from build123d import *

# Parameters (mm, degrees)
F1_DEPTH = 38.1
F3_DEPTH = 12.7
F5_DEPTH = 12.7
F6_DEPTH = 25.4
F8_DEPTH = 12.7


with BuildPart() as f1:
    # F0 (on Front) → F1 (new body)
    with BuildSketch(Plane.XZ):
        Polygon((0, 12.7), (0, 0), (25.4, 0), (25.4, 38.1), (12.7, 38.1), (12.7, 12.7), align=None)
    extrude(amount=F1_DEPTH)

    # F2 (on face) → F3 (cut)
    with BuildSketch(Plane(origin=(12.7, 0, 0), x_dir=(0, -1, 0), z_dir=(-1, 0, 0))):
        Polygon((38.1, 38.1), (25.4, 38.1), (38.1, 12.7), align=None)
    extrude(amount=-F3_DEPTH, mode=Mode.SUBTRACT)

    # F4 (on face) → F5 (join)
    with BuildSketch(Plane.XY.offset(12.7)):
        Polygon((0, -38.1), (12.7, -38.1), (0, -31.632963568), align=None)
    extrude(amount=F5_DEPTH)

    # F6 (cut): a face of the model
    f6_faces = [f1.faces().sort_by_distance(p)[0] for p in [
        (6.35, -34.866481784, 19.05),
    ]]
    extrude(f6_faces, amount=-F6_DEPTH, mode=Mode.SUBTRACT)

    # F7 (on face) → F8 (cut)
    with BuildSketch(Plane.XY.offset(12.7)):
        Polygon((12.7, -38.1), (0, -29.6376030892), (0, -38.1), align=None)
    extrude(amount=-F8_DEPTH, mode=Mode.SUBTRACT)


solid = f1.part
For this review, take the finished solid that the model builds, in its own axes (mm). A direction names the side the tool comes from. Round coordinates to 2 decimals unless told otherwise and drop trailing zeros. Order: outer loops, then holes, each group sorted by start corner. A loop starts at its lowest first (then second) coordinate and runs counter-clockwise, first axis right, second up. Notation, with made-up numbers: (27, -20) -> (49, -20) arc R27 ccw to (49, 4) -> close; hole circle Ø9 at (40.25, -39). An arc over 180 degrees is marked (long way). Write item = value, one per line. Start each with the question number.
1) Tool access review of faces 4 (the face through (13, -19, 0)), 5 (the face through (8, -16, 12.7)): name each direction out of +Z, -Z, +X, -X, +Y, -Y from which nothing blocks a thin tool from reaching the whole face with its end or side.
2) Take a section at A-A on y = -13.5. State the section outline as (x, z) points.
3) Take a section at B-B on z = 6.5. State the section outline as (x, y) points, plus the area to 3 significant figures.
4) The part is to be moulded in two halves that separate along X. For faces 1 (the face through (25.4, -19, 19)), 2 (the face through (19, -38.1, 6)), 3 (the face through (6.4, -33.9, 6.4)), say which applies: +X half, -X half, draft (parallel to the pull), parting line (faces both ways), or undercut.
5) Take a section at C-C on x = 14.75. State the section outline as (y, z) points, plus the area to 3 significant figures.
6) Insertion check: pin 1 (5 mm diameter, centred on y = -26, z = 32, fed in from -X); pin 2 (8 mm diameter, centred on x = 15.5, y = -33.5, fed in from +Z); pin 3 (6.5 mm diameter, centred on x = 9, y = -20, fed in from +Z). Each pin has a flat end and moves straight along its axis. Give the tip position at first contact, or say it passes through.
7) Take a section at D-D on y = -26.5. State the section outline as (x, z) points.
8) To check wall thickness, follow line 1 (X direction, y = -16.5, z = 29.5); line 2 (Z direction, x = 11.5, y = -25); line 3 (Y direction, x = 6.5, z = 8.5). State the ranges of each line that lie inside material, in increasing order. Write a range as from..to.
Verdict:
q1.face_4 = -Z, +X, -X, +Y, -Y
q1.face_5 = +Z, -X, +Y, -Y
q2.outline = (0, 0) -> (25.4, 0) -> (25.4, 38.1) -> (12.7, 38.1) -> (12.7, 12.7) -> (0, 12.7) -> close
q3.outline = (0, -29.64) -> (12.7, -38.1) -> (25.4, -38.1) -> (25.4, 0) -> (0, 0) -> close
q3.area = 914 mm2
q4.face_1 = +X half
q4.face_2 = draft
q4.face_3 = -X half
q5.outline = (-38.1, 0) -> (0, 0) -> (0, 38.1) -> (-25.4, 38.1) -> (-38.1, 12.7) -> close
q5.area = 1,290 mm2
q6.pin_1 = 12.7
q6.pin_2 = 29.9
q6.pin_3 = 12.7
q7.outline = (0, 0) -> (25.4, 0) -> (25.4, 35.9) -> (12.7, 35.9) -> (12.7, 12.7) -> (0, 12.7) -> close
q8.line_1 = 12.7..25.4
q8.line_2 = 0..12.7
q8.line_3 = -33.97..0
